```python
from build123d import *

# Parameters (mm, degrees)
BOX001_W     = 35
BOX001_H     = 70
BOX001_DEPTH = 9
BOX_W        = 38
BOX_H        = 73
BOX_DEPTH    = 10
FILLET_R     = 2


with BuildPart() as interior:
    # Box001 → Box001 (new body)
    with BuildSketch(Plane(origin=(1.5, 1.5, 1.5), x_dir=(1, 0, 0), z_dir=(0, 0, 1))):
        with Locations((17.5, 35)):
            Rectangle(BOX001_W, BOX001_H)
    extrude(amount=BOX001_DEPTH)


with BuildPart() as obj1:
    # Box → Box (new body)
    with BuildSketch(Plane.XY):
        with Locations((19, 36.5)):
            Rectangle(BOX_W, BOX_H)
    extrude(amount=BOX_DEPTH)

    # Cut: cut Interior
    add(interior.part, mode=Mode.SUBTRACT)

    # Fillet
    fillet_edges = [obj1.edges().sort_by_distance(p)[0] for p in [
        (0, 0, 5),
        (0, 73, 5),
        (38, 0, 5),
        (38, 73, 5),
    ]]
    fillet(fillet_edges, radius=FILLET_R)


solid = obj1.part
```
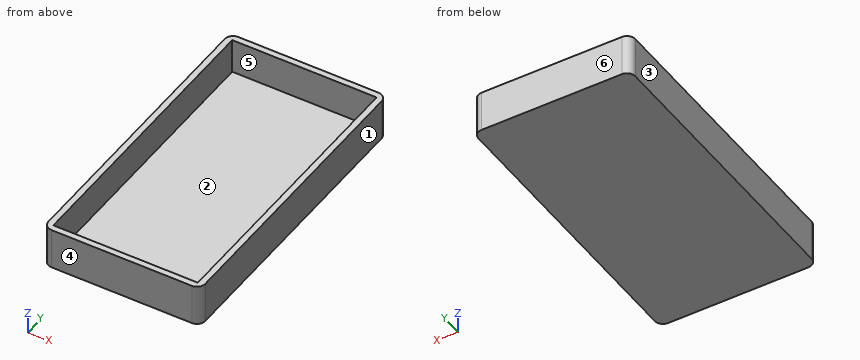
CAD build for the part. Positions are in the model's coordinates, mm. Face numbers are marked on the shaded views. A direction names the side the tool comes from. Coordinates: 2 decimals unless noted, no trailing zeros. Write each loop counter-clockwise with the first axis right and the second up, starting at its lowest first coordinate (ties: lowest second). Pieces come first, ordered by that corner, then holes.
(1) 3-axis set-ups, long thin cutter, end or side, ignore diameter. For the marked faces 5 and 6: which of +Z, -Z, +X, -X, +Y, -Y reach the whole face in a straight line?
(2) Drill centre lines: probe 1 along Y at (x, z) = (21, 6.5); probe 2 along X at (y, z) = (53.5, 7.5); probe 3 along Z at (x, y) = (13, 23.5). Where is each one in solid material? Low to high.
(3) Cut at A-A, the plane z = 7.25. List the corners of the cut face in (x, y).
(4) Two-plate mould, pull along X, no slides. Class the marked faces 1, 2, 3 and 4: +X half, -X half, draft (parallel to the pull), parting line (faces both ways), or undercut.
(5) Cut at C-C, the plane x = 9.5. List the corners of the cut face in (y, z), and give its area (3 significant figures).
(6) Flat gauge pin, fed straight in: pin 1 (3 mm diameter, centred on x = 7.5, y = 57.5, fed in from +Z). Where does the tip first touch, or does it go through?
(7) Cut at B-B, the plane y = 36. List the corners of the cut face in (x, z).
Geometry says:
1. face 5: +Z
1. face 6: +Z, -Z, +X, -X, +Y
2. probe 1: y = 0 to 1.5, 71.5 to 73
2. probe 2: x = 0 to 1.5, 36.5 to 38
2. probe 3: z = 0 to 1.5
3. outline: (0, 2) arc R2 ccw to (2, 0) - (36, 0) arc R2 ccw to (38, 2) - (38, 71) arc R2 ccw to (36, 73) - (2, 73) arc R2 ccw to (0, 71) - close; hole (1.5, 1.5) - (36.5, 1.5) - (36.5, 71.5) - (1.5, 71.5) - close
4. face 1: +X half
4. face 2: undercut
4. face 3: -X half
4. face 4: draft
5. outline: (0, 0) - (73, 0) - (73, 10) - (71.5, 10) - (71.5, 1.5) - (1.5, 1.5) - (1.5, 10) - (0, 10) - close
5. area: 135 mm2
6. pin 1: stops at z = 1.5
7. outline: (0, 0) - (38, 0) - (38, 10) - (36.5, 10) - (36.5, 1.5) - (1.5, 1.5) - (1.5, 10) - (0, 10) - close
